Read the model definition and answer for the solid it produces. Units are mm, in the model's axes. Give positions to 0.01 mm unless a question says otherwise; leave off trailing zeros. Loops run counter-clockwise (first coordinate to the right, second up) from the corner with the lowest first, then second, coordinate; pieces in that order, holes last. Notation, with made-up numbers: (-11, 40) - (40, 40) arc R19 cw to (40, 51) - close; hole circle Ø11 at (-35.75, 83). An arc over 180 degrees is marked (long way). Write item = value, one per line.
```python
from build123d import *

# Parameters (mm, degrees)
SKETCH_1_W          = 41
SKETCH_1_H          = 41
SKETCH_1_R          = 11
EXTRUDE_1_DEPTH     = 3
SKETCH_4_R          = 2.25
CUT_EXTRUDE_2_DEPTH = 4
CHAMFER_1_SIZE      = 2.5


with BuildPart() as part:
    # Эскиз1 → Вытянуть1 (new body)
    with BuildSketch(Plane.XY):
        Rectangle(SKETCH_1_W, SKETCH_1_H)
        Circle(SKETCH_1_R, mode=Mode.SUBTRACT)
    extrude(amount=EXTRUDE_1_DEPTH)

    # Эскиз4 → Вытянуть2 (cut, through all)
    with BuildSketch(Plane.XY.offset(3)):
        with Locations((-14.495689014, 14.495689014)):
            Circle(SKETCH_4_R)
        with Locations((14.495689014, 14.495689014)):
            Circle(SKETCH_4_R)
        with Locations((14.495689014, -14.495689014)):
            Circle(SKETCH_4_R)
        with Locations((-14.495689014, -14.495689014)):
            Circle(SKETCH_4_R)
    extrude(amount=-CUT_EXTRUDE_2_DEPTH, mode=Mode.SUBTRACT)

    # Фаска1
    chamfer_1_edges = [part.edges().sort_by_distance(p)[0] for p in [
        (20.5, -20.5, 1.5),
        (-20.5, -20.5, 1.5),
        (-20.5, 20.5, 1.5),
        (20.5, 20.5, 1.5),
    ]]
    chamfer(chamfer_1_edges, length=CHAMFER_1_SIZE)


solid = part.part
```
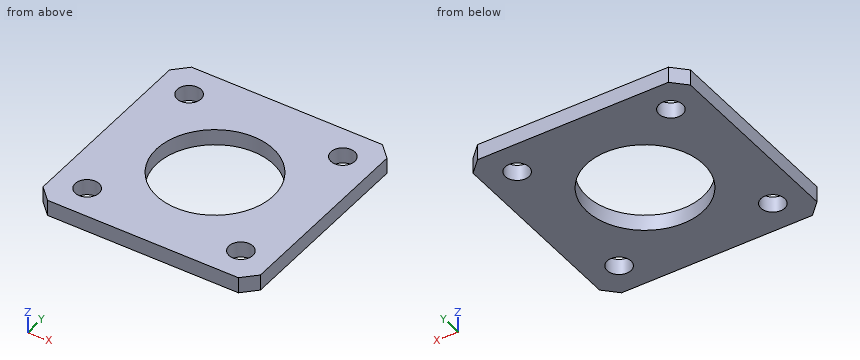
1) A cutting plane is placed at D-D on y = 15.5. Determine the outline of the cut face in (x, z), then the cut area to 3 significant figures.
Output:
outline = (-20.5, 0) - (-16.51, 0) - (-16.51, 3) - (-20.5, 3) - close; (-12.48, 0) - (12.48, 0) - (12.48, 3) - (-12.48, 3) - close; (16.51, 0) - (20.5, 0) - (20.5, 3) - (16.51, 3) - close
area = 98.8 mm²
2) Find the intervals of material crossed by probe 1 along Y at (x, z) = (16, 2.8); probe 2 along Y at (x, z) = (0, 0.6); probe 3 along X at (y, z) = (-2, 1.6), in increasing order.
Output:
probe_1 = -20.5 to -16.17, -12.82 to 12.82, 16.17 to 20.5
probe_2 = -20.5 to -11, 11 to 20.5
probe_3 = -20.5 to -10.82, 10.82 to 20.5
3) A cutting plane is placed at A-A on x = 0. Determine the outline of the cut face in (y, z).
Output:
outline = (-20.5, 0) - (-11, 0) - (-11, 3) - (-20.5, 3) - close; (11, 0) - (20.5, 0) - (20.5, 3) - (11, 3) - close
4) This flat-tipped pin is pushed along its axis until it touches: P1, Ø5, axis at x = -14.5, y = -14.5, coming from the +Z side. Where does it stop, or does it pass through?
Output:
P1 = 3
5) A cutting plane is placed at C-C on z = 2.2. Determine the outline of the cut face in (x, y), then the cut area to 3 significant figures.
Output:
outline = (-20.5, -18) - (-18, -20.5) - (18, -20.5) - (20.5, -18) - (20.5, 18) - (18, 20.5) - (-18, 20.5) - (-20.5, 18) - close; hole circle Ø4.5 at (-14.5, -14.5); hole circle Ø4.5 at (-14.5, 14.5); hole circle Ø22 at (0, 0); hole circle Ø4.5 at (14.5, -14.5); hole circle Ø4.5 at (14.5, 14.5)
area = 1,220 mm²
